from build123d import *

# Parameters (mm, degrees)
F3_D     = 8
F5_DEPTH = 12.5
F7_DEPTH = 12.5


with BuildPart() as f1:
    # F0 (on Front) → F1 (revolve)
    with BuildSketch(Plane.XZ):
        Polygon((-15, 0), (0, 0), (0, 35), (-6, 35), (-6, 10), (-15, 10), align=None)
    revolve(axis=Axis((0, 0, 17.5), (0, 0, 1)))

    # F3 (through all)
    with Locations(Plane(origin=(0, 0, 0), x_dir=(1, 0, 0), z_dir=(0, 0, -1))):
        with Locations((0, 0)):
            Hole(F3_D / 2)

    # F4 (on Front) → F5 (cut, symmetric)
    with BuildSketch(Plane.XZ):
        Polygon((-1.5, 10), (0, 10), (1.5, 10), (1.5, 35), (0, 35), (-1.5, 35), align=None)
    extrude(amount=F5_DEPTH, both=True, mode=Mode.SUBTRACT)

    # F6 (on Right) → F7 (cut, symmetric)
    with BuildSketch(Plane.YZ):
        Polygon((-1.5, 10), (0, 10), (1.5, 10), (1.5, 35.1293485655), (0, 35.1293485655), (-1.5, 35.1293485655), align=None)
    extrude(amount=F7_DEPTH, both=True, mode=Mode.SUBTRACT)


solid = f1.part
The listing builds one solid part. Answer for the finished solid, in the listing's coordinates (mm). A direction names the side the tool comes from. Round coordinates to 2 decimals unless told otherwise and drop trailing zeros. Loops run counter-clockwise (first coordinate to the right, second up) from the corner with the lowest first, then second, coordinate; pieces in that order, holes last. Notation, with made-up numbers: M 10,6.5 L 22,6.5 A20 cw 22,18.5 Z; hole C -35,-5 d3. An arc over 180 degrees is marked long. Write each question's results on one line, items separated by ' | '. Start each with the question number.
1) Find section D-D on z = 8. Write down the section's boundary in (x, y), plus the area to 3 significant figures.
2) Straight lines are drawn through the part: probe 1 along Y at (x, z) = (0, 8); probe 2 along Y at (x, z) = (-3.5, 32); probe 3 along Z at (x, y) = (7.75, 3.25). For each, find the intervals that lie inside material, in ascending order.
3) Find section A-A on x = 0. Write down the section's boundary in (y, z), plus the area to 3 significant figures.
4) Find section C-C on z = 13. Write down the section's boundary in (x, y).
5) Which of the six approach directions +Z, -Z, +X, -X, +Y, -Y give full straight-line access (tool end or side, diameter ignored) to faces 4 (the flat face through (5, 1.5, 22)), 5 (the flat face through (1.5, -5, 22)), 6 (the cylindrical face through (4.211, -4.274, 22.325))?
6) Determine the mould class of faces 1 (the flat face through (-3, 3, 0)), 2 (the cylindrical face through (-4.274, -4.211, 22.325)), 3 (the flat face through (-5, -1.5, 23)) for opening direction Y: pulls with the +Y half, pulls with the -Y half, needs draft (parallel to the pull), parting line crosses it, or undercut.
7) Each of these flat-tipped pins is pushed along its axis until it touches: pin 1 (1.7 mm diameter, centred on y = -5, z = 24.5, fed in from +X); pin 2 (8 mm diameter, centred on y = 0, z = 16.5, fed in from -X); pin 3 (1 mm diameter, centred on x = -1.5, y = 7, fed in from +Z). Where does it stop, or does it pass through?
Final values:
1) outline: C 0,0 d30; hole C 0,0 d8 | area: 657 mm²
2) probe 1: -15 to -4, 4 to 15 | probe 2: -4.87 to -1.94, 1.94 to 4.87 | probe 3: 0 to 10
3) outline: M -15,0 L -4,0 L -4,10 L -15,10 Z; M 4,0 L 15,0 L 15,10 L 4,10 Z | area: 220 mm²
4) outline: M -5.81,-1.5 A6 ccw -1.5,-5.81 L -1.5,-3.71 A4 cw -3.71,-1.5 Z; M -5.81,1.5 L -3.71,1.5 A4 cw -1.5,3.71 L -1.5,5.81 A6 ccw Z; M 1.5,-5.81 A6 ccw 5.81,-1.5 L 3.71,-1.5 A4 cw 1.5,-3.71 Z; M 1.5,3.71 A4 cw 3.71,1.5 L 5.81,1.5 A6 ccw 1.5,5.81 Z
5) face 4: +Z, +X, -X | face 5: +Z, +Y, -Y | face 6: +Z, +X, -Y
6) face 1: needs draft | face 2: pulls with the -Y half | face 3: undercut
7) pin 1: x = 4.33 | pin 2: x = -5.81 | pin 3: z = 10
